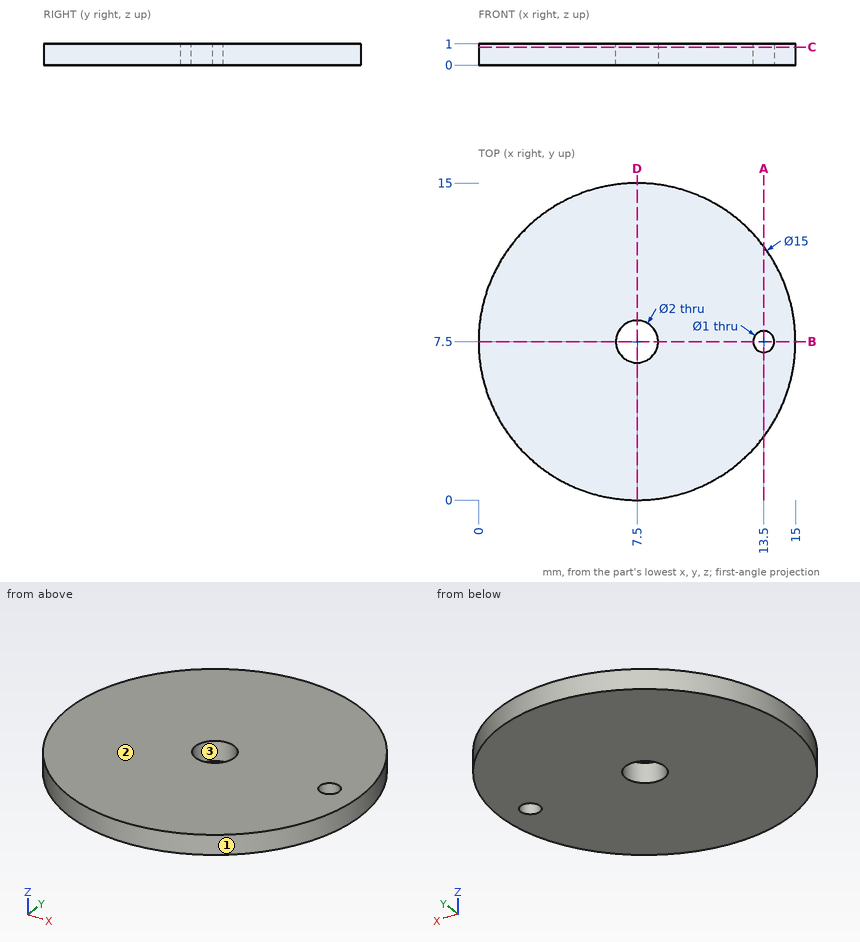
Answer from the drawing. Dimensions are ordinates in mm from the lowest x, y and z of the part. Give positions to 0.01 mm unless a question says otherwise; leave off trailing zeros. Write each loop counter-clockwise with the first axis right and the second up, starting at its lowest first coordinate (ties: lowest second). Pieces come first, ordered by that corner, then holes.
1) Section D-D (x = 7.5) is taken. Write down the section's boundary in (y, z), and give its area (3 significant figures).
2) Find the intervals of material crossed by L1, parallel to Y at x = 7.5, z = 0.3; L2, parallel to Y at x = 7, z = 0.55; L3, parallel to X at y = 7.25, z = 0.8, in increasing order.
3) Section B-B (y = 7.5) is taken. Write down the section's boundary in (x, z), and give its area (3 significant figures).
4) Section A-A (x = 13.5) is taken. Write down the section's boundary in (y, z), and give its area (3 significant figures).
5) Given P1, Ø8, axis at x = 5.5, y = 2.5, coming from the -Z side, flat-ended and moving along its own axis, determine where the tip first touches the part or whether it passes through.
6) Section C-C (z = 0.85) is taken. Write down the section's boundary in (x, y).
7) For a pull along X with two mould halves and no side action, classify the marked faces 1, 2 and 3 as pulls with the +X half, pulls with the -X half, needs draft (parallel to the pull), parting line crosses it, or undercut.
Response:
1. outline: (0, 0) - (6.5, 0) - (6.5, 1) - (0, 1) - close; (8.5, 0) - (15, 0) - (15, 1) - (8.5, 1) - close
1. area: 13.0 mm2
2. L1: y = 0 to 6.5, 8.5 to 15
2. L2: y = 0.02 to 6.63, 8.37 to 14.98
2. L3: x = 0 to 6.53, 8.47 to 13.07, 13.93 to 15
3. outline: (0, 0) - (6.5, 0) - (6.5, 1) - (0, 1) - close; (8.5, 0) - (13, 0) - (13, 1) - (8.5, 1) - close; (14, 0) - (15, 0) - (15, 1) - (14, 1) - close
3. area: 12.0 mm2
4. outline: (3, 0) - (7, 0) - (7, 1) - (3, 1) - close; (8, 0) - (12, 0) - (12, 1) - (8, 1) - close
4. area: 8.00 mm2
5. P1: stops at z = 0
6. outline: circle Ø15 at (7.5, 7.5); hole circle Ø2 at (7.5, 7.5); hole circle Ø1 at (13.5, 7.5)
7. face 1: parting line crosses it
7. face 2: needs draft
7. face 3: undercut
